```python
from build123d import *

# Parameters (mm, degrees)
CROQUIS1_R              = 13.7
CROQUIS2_W              = 104.810760898
CROQUIS2_H              = 208.017118972
CORTAR_EXTRUIR2_DEPTH   = 81
CROQUIS3_R              = 17.762543943
CROQUIS3_R_2            = 15
SALIENTE_EXTRUIR1_DEPTH = 10
CROQUIS4_W              = 40.294914154
CROQUIS4_H              = 26.389647966
SALIENTE_EXTRUIR2_DEPTH = 10


with BuildPart() as part:
    # Barrer1: sweep along a curve in space
    with BuildLine() as barrer1_path:
        Line((0, 0, 0), (-30, 0, 0))
        ThreePointArc((-30, 0, 0), (-44.142135624, 5.857864376, 0), (-50, 20, 0))
        Line((-50, 20, 0), (-50, 100, 0))
        ThreePointArc((-50, 100, 0), (-55.857864376, 114.142135624, 0), (-70, 120, 0))
        Line((-70, 120, 0), (-230, 120, 0))
        ThreePointArc((-230, 120, 0), (-244.142135624, 125.857864376, 0), (-250, 140, 0))
        Line((-250, 140, 0), (-250, 890, 0))
        ThreePointArc((-250, 890, 0), (-250, 904.142135624, 5.857864376), (-250, 910, 20))
        Line((-250, 910, 20), (-250, 910, 80))
        ThreePointArc((-250, 910, 80), (-250, 915.857864376, 94.142135624), (-250, 930, 100))
        Line((-250, 930, 100), (-250, 940, 100))
        ThreePointArc((-250, 940, 100), (-250, 954.142135624, 105.857864376), (-250, 960, 120))
        Line((-250, 960, 120), (-250, 960, 150))
    # Croquis1 → Barrer1 (sweep)
    with BuildSketch(Plane(origin=(0, 0, 0), x_dir=(0, 0, -1), z_dir=(1, 0, 0))):
        Circle(CROQUIS1_R)
    sweep(path=barrer1_path.line)

    # Croquis2 → Cortar-Extruir2 (cut)
    with BuildSketch(Plane.XY.offset(150)):
        with Locations((-250, 960)):
            Rectangle(CROQUIS2_W, CROQUIS2_H)
    extrude(amount=-CORTAR_EXTRUIR2_DEPTH, mode=Mode.SUBTRACT)



with BuildPart() as body_2:
    # Croquis3 → Saliente-Extruir1 (new body)
    with BuildSketch(Plane(origin=(0, 0, 0), x_dir=(1, 0, 0), z_dir=(0, 1, 0))):
        with Locations((35, 0)):
            Circle(CROQUIS3_R)
        with Locations((35, 0)):
            Circle(CROQUIS3_R_2, mode=Mode.SUBTRACT)
    extrude(amount=SALIENTE_EXTRUIR1_DEPTH)


with BuildPart() as part_1:
    add(part.part)

    add(body_2.part)  # Saliente-Extruir2 merges body 2
    # Croquis4 → Saliente-Extruir2 (add)
    with BuildSketch(Plane(origin=(0, 0, 0), x_dir=(1, 0, 0), z_dir=(0, 1, 0))):
        Rectangle(CROQUIS4_W, CROQUIS4_H)
    extrude(amount=SALIENTE_EXTRUIR2_DEPTH)


solid = part_1.part
```
Can you work these out from the model? Positions are in its coordinate system, mm. A direction names the side the tool comes from. Coordinates: 2 decimals unless noted, no trailing zeros. Loops run counter-clockwise (first coordinate to the right, second up) from the corner with the lowest first, then second, coordinate; pieces in that order, holes last.
Item 1: Suppose I cut it at C-C (y = 294). Please give me the cut outline in (x, z), then the cut area to 3 significant figures.
Answers below:
outline: circle Ø27.4 at (-250, 0)
area: 590 mm2
Item 2: Please list where these lines run through material, in increasing order: L1, parallel to Y at x = -25, z = 1; L2, parallel to X at y = 650.5, z = 8; L3, parallel to Y at x = -159, z = -3.5.
Answers below:
L1: y = -13.66 to 13.66
L2: x = -261.12 to -238.88
L3: y = 106.75 to 133.25
Item 3: Suppose I cut it at A-A (x = 35). Please give me the cut outline in (y, z), then the cut area to 3 significant figures.
Answers below:
outline: (0, -17.76) - (10, -17.76) - (10, -15) - (0, -15) - close; (0, 15) - (10, 15) - (10, 17.76) - (0, 17.76) - close
area: 55.3 mm2
Item 4: I'm going to push flat-ended pins straight in: pin 1 (1.7 mm diameter, centred on y = 5, z = -12, fed in from +X); pin 2 (1.5 mm diameter, centred on y = 161, z = 5, fed in from -X); pin 3 (5 mm diameter, centred on x = -2, y = 4.5, fed in from +Z); pin 4 (10.5 mm diameter, centred on x = 29, z = 3.5, fed in from -Y). Where does each tip first touch, or does it pass through?
Answers below:
pin 1: stops at x = 48.83
pin 2: stops at x = -263.02
pin 3: stops at z = 13.55
pin 4: passes through
Item 5: Which directions (+Z, -Z, +X, -X, +Y, -Y) give clear straight access to the entire face, cutting with the end or side of a thin tool? Please do faces 1 (the face through (-254.115, 923.067, 44.843)), 2 (the face through (14, 0, 0)), 3 (the face through (-263.583, 520.25, 1.783)).
Answers below:
face 1: +Z
face 2: +Z, -Z, +X, -Y
face 3: none
Item 6: Suppose I cut it at B-B (z = 37.5). Please give me the cut outline in (x, y).
Answers below:
outline: circle Ø27.4 at (-250, 910)
